Verification items for this drawing (mm, ordinates from the low corner). A direction names the side the tool comes from. Round coordinates to 2 decimals unless told otherwise and drop trailing zeros. Write each loop counter-clockwise with the first axis right and the second up, starting at its lowest first coordinate (ties: lowest second). Pieces come first, ordered by that corner, then holes. Notation, with made-up numbers: M 38.25,74.25 L 54.25,74.25 A24 cw 54.25,107.25 Z; hole C 28.5,-27 d6. An arc over 180 degrees is marked long. One line per question, with ' | ' between items. Start each with the question number.
Q1. Cross-section at C-C (x = 1.75). Record the boundary of the cut face in (y, z), then the cut area to 3 significant figures.
Q2. Cross-section at A-A (y = 80.5). Record the boundary of the cut face in (x, z), then the cut area to 3 significant figures.
Q3. Gauge pin test, flat ends, axial feed: pin 1 (3 mm diameter, centred on x = 17, y = 53.5, fed in from -Z); pin 2 (5 mm diameter, centred on x = 2, y = 40, fed in from -Z); pin 3 (1.3 mm diameter, centred on x = 15, z = 18.5, fed in from -Y). Record the tip position at first contact, or that the pin passes through.
Q4. Thickness scan on line 1 along X through (y, z) = (63, 12.75); line 2 along X through (y, z) = (73.5, 5); line 3 along Y through (x, z) = (14.25, 19). Record the ranges inside material, lowest first. Write a range as from..to.
Q5. Tool access check on the marked faces 1, 2 and 3. Record the directions out of +Z, -Z, +X, -X, +Y, -Y that give a thin tool (end or side, any length) a straight path to the whole face; none if there is none.
Q6. Cross-section at D-D (z = 12.5). Record the boundary of the cut face in (x, y).
Q7. Cross-section at B-B (z = 17). Record the boundary of the cut face in (x, y), then the cut area to 3 significant figures.
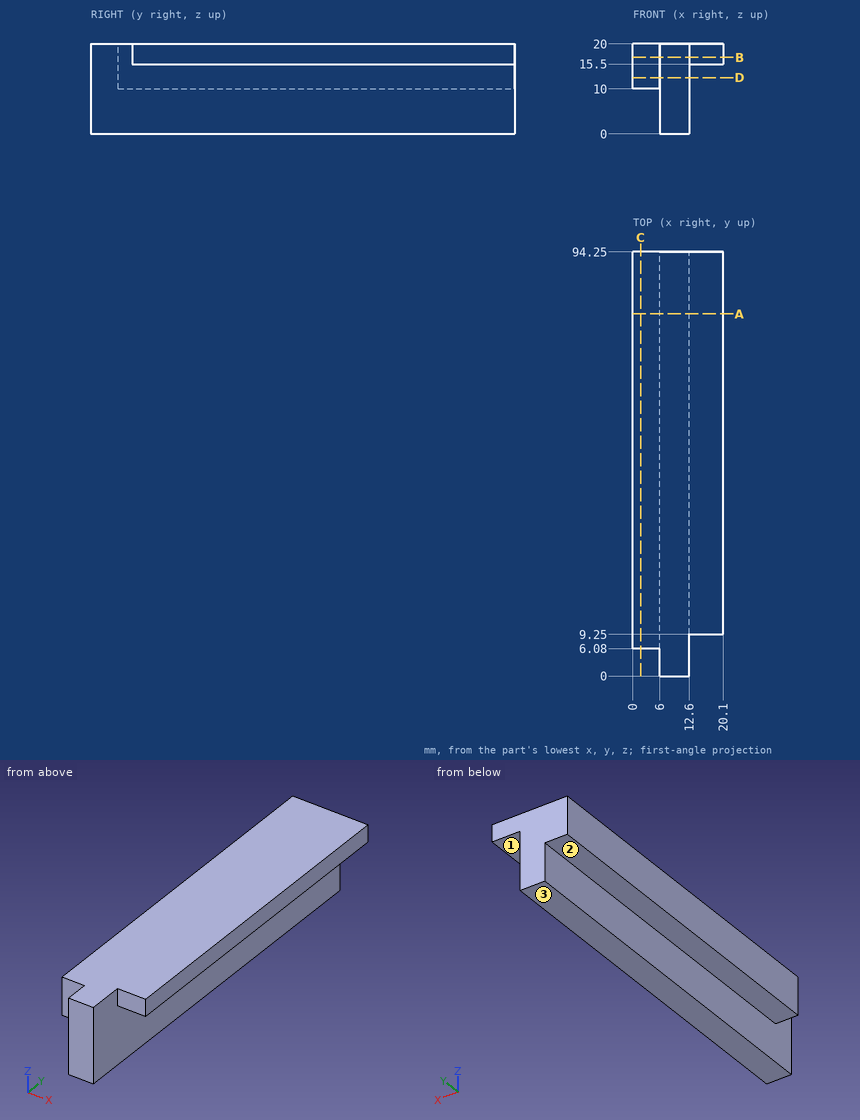
Determined:
1) outline: M 6.08,10 L 94.25,10 L 94.25,20 L 6.08,20 Z | area: 882 mm²
2) outline: M 0,10 L 6,10 L 6,0 L 12.6,0 L 12.6,15.5 L 20.1,15.5 L 20.1,20 L 0,20 Z | area: 226 mm²
3) pin 1: stops at z = 15.5 | pin 2: stops at z = 10 | pin 3: stops at y = 9.25
4) line 1: x = 0..12.6 | line 2: x = 6..12.6 | line 3: y = 9.25..94.25
5) face 1: -Z, +X, +Y, -Y | face 2: -Z, -X, +Y, -Y | face 3: -Z, +X, -X, +Y, -Y
6) outline: M 0,6.08 L 6,6.08 L 6,0 L 12.6,0 L 12.6,94.25 L 0,94.25 Z
7) outline: M 0,6.08 L 6,6.08 L 6,0 L 12.6,0 L 12.6,9.25 L 20.1,9.25 L 20.1,94.25 L 0,94.25 Z | area: 1,790 mm²
